Geometry check sheet. Reference: drawing and pictorial views, mm from the part's lowest x, y, z. Coordinates: 2 decimals unless noted, no trailing zeros. Write each loop counter-clockwise with the first axis right and the second up, starting at its lowest first coordinate (ties: lowest second). Pieces come first, ordered by that corner, then holes. Notation, with made-up numbers: (81.5, 16) -> (133.5, 16) arc R26 ccw to (133.5, 36) -> close; hole circle Ø1 at (47.25, 80.5). An arc over 180 degrees is marked (long way). Answer in a Markdown table with one row per item.
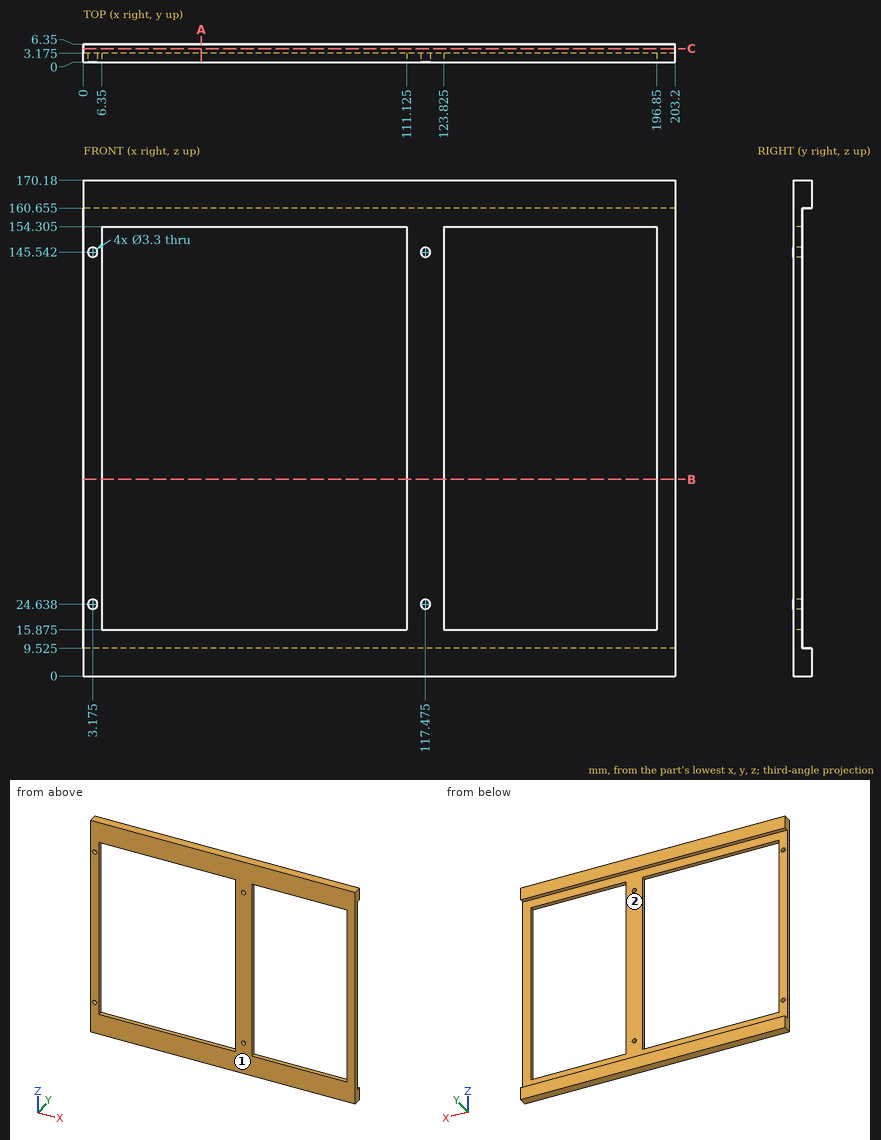
1. Mould release check, pull along Z, two halves, no side actions. Record for the marked faces 1 and 2: released by +Z, released by -Z, zero draft, split by the parting line, or undercut.
Geometry says:
| item | result |
|---|---|
| face 1 | zero draft |
| face 2 | undercut |
2. Thickness scan on line 1 (Z direction, x = 18.5, y = 2) (3 decimals); line 2 (Z direction, x = 160, y = 6.25) (3 decimals); line 3 (Y direction, x = 147, z = 160) (3 decimals). Record the ranges inside material, lowest first. Write a range as from..to.
Geometry says:
| item | result |
|---|---|
| line 1 | 0..15.875, 154.305..170.18 |
| line 2 | 0..9.525, 160.655..170.18 |
| line 3 | 0..3.175 |
3. Section check C-C, the plane y = 4.75. Record the boundary of the cut face in (x, z) (3 decimals).
Geometry says:
| item | result |
|---|---|
| outline | (0, 0) -> (203.2, 0) -> (203.2, 9.525) -> (0, 9.525) -> close; (0, 160.655) -> (203.2, 160.655) -> (203.2, 170.18) -> (0, 170.18) -> close |
4. Depth check by flat-ended pin: P1, Ø2.5, axis at x = 3.175, z = 24.638, coming from the -Y side. Enter the tip coordinate at first touch or a pass-through.
Geometry says:
| item | result |
|---|---|
| P1 | through |
5. Section check A-A, the plane x = 40.5. Record the boundary of the cut face in (y, z) (3 decimals).
Geometry says:
| item | result |
|---|---|
| outline | (0, 0) -> (6.35, 0) -> (6.35, 9.525) -> (3.175, 9.525) -> (3.175, 15.875) -> (0, 15.875) -> close; (0, 154.305) -> (3.175, 154.305) -> (3.175, 160.655) -> (6.35, 160.655) -> (6.35, 170.18) -> (0, 170.18) -> close |
6. Section check B-B, the plane z = 67.5. Record the boundary of the cut face in (x, y) (3 decimals), plus the area to 3 significant figures.
Geometry says:
| item | result |
|---|---|
| outline | (0, 0) -> (6.35, 0) -> (6.35, 3.175) -> (0, 3.175) -> close; (111.125, 0) -> (123.825, 0) -> (123.825, 3.175) -> (111.125, 3.175) -> close; (196.85, 0) -> (203.2, 0) -> (203.2, 3.175) -> (196.85, 3.175) -> close |
| area | 80.6 mm^2 |
